from build123d import *

# Parameters (mm, degrees)
EXTRUDE_THIN1_DEPTH = 349.25
FILLET1_R           = 1.016


with BuildPart() as part:
    # Sketch1 → Extrude-Thin1 (new body)
    with BuildSketch(Plane.XY):
        with BuildLine():
            Line((0, 34.925), (-14.2875, 34.925))
            Line((-14.2875, 34.925), (-14.2875, 23.8125))
            Line((-14.2875, 23.8125), (-12.7, 23.8125))
            ThreePointArc((-12.7, 23.8125), (-11.46897023, 18.728780658), (-8.048625, 14.771398298))
            ThreePointArc((-8.048625, 14.771398298), (-4.62827977, 10.814015938), (-3.39725, 5.730296596))
            Line((-3.39725, 5.730296596), (-1.016, 5.730296596))
            Line((-1.016, 5.730296596), (-1.016, 4.7625))
            ThreePointArc((-1.016, 4.7625), (-3.39725, 2.38125), (-1.016, 0))
            Line((-1.016, 0), (0, 0))
            Line((0, 0), (0, 1.016))
            Line((0, 1.016), (-1.016, 1.016))
            ThreePointArc((-1.016, 1.016), (-2.26278514, 2.93751826), (0, 3.29319932))
            Line((0, 3.29319932), (0, 6.746296596))
            Line((0, 6.746296596), (-2.423879893, 6.746296596))
            ThreePointArc((-2.423879893, 6.746296596), (-3.966915161, 11.726057249), (-7.457893571, 15.598013311))
            ThreePointArc((-7.457893571, 15.598013311), (-10.786815308, 19.651741643), (-11.632750432, 24.8285))
            Line((-11.632750432, 24.8285), (-13.2715, 24.8285))
            Line((-13.2715, 24.8285), (-13.2715, 33.909))
            Line((-13.2715, 33.909), (0, 33.909))
            Line((0, 33.909), (0, 34.925))
        make_face()
    extrude(amount=-EXTRUDE_THIN1_DEPTH)

    # Fillet1
    fillet1_edges = [part.edges().sort_by_distance(p)[0] for p in [
        (-11.632750432, 24.8285, -174.625),
        (0, 6.746296596, -174.625),
        (0, 3.29319932, -174.625),
        (-3.39725, 5.730296596, -174.625),
        (-14.2875, 23.8125, -174.625),
        (-14.2875, 34.925, -174.625),
    ]]
    fillet(fillet1_edges, radius=FILLET1_R)


solid = part.part
Build history of the part. All positions in model axes, mm. A direction names the side the tool comes from. Give positions to 0.01 mm unless a question says otherwise; leave off trailing zeros. Write each loop counter-clockwise with the first axis right and the second up, starting at its lowest first coordinate (ties: lowest second). Pieces come first, ordered by that corner, then holes. Notation, with made-up numbers: (35.5, 54.25) - (91.5, 54.25) arc R21 cw to (91.5, 58.25) - close; hole circle Ø8 at (-23.75, 69.5). An arc over 180 degrees is marked (long way). Use one line per item in the form item = value. Start each with the question number.
1. 3-axis set-ups, long thin cutter, end or side, ignore diameter. For faces 5 (the face through (-3.93, 11.66, -172.18)), 6 (the face through (-11.4, 20.1, -349.25)): which of +Z, -Z, +X, -X, +Y, -Y reach the whole face in a straight line?
2. Band-saw the part on B-B on y = 31. Write the cut outline in (x, z).
3. Two-plate mould, pull along Y, no slides. Class faces 1 (the face through (-14.288, 29, -172)), 2 (the face through (-10.535, 19.134, -172.18)), 3 (the face through (-7, 34.925, -172)), 4 (the face through (-13.272, 29, -172)): released by +Y, released by -Y, zero draft, split by the parting line, or undercut.
4. Band-saw the part on A-A on z = -249.5. Write the cut outline in (x, y) (1 decimal).
5. Band-saw the part on C-C on y = 18.5. Write the cut outline in (x, z).
6. Probe line 1 (X direction, y = 32.5, z = -237); line 2 (Y direction, x = -6.5, z = -176) (3 decimals); line 3 (Y direction, x = -5.25, z = -330) (3 decimals). List the from-to ranges inside material, lowest first. Write a range as [from, to].
7. Drop flat-ended pins along their axis: pin 1 Ø3 at (x, y) = (-7, 18.5) entering from -Z; pin 2 Ø1.1 at (y, z) = (5, -225) entering from -X; pin 3 Ø2 at (x, z) = (-12, -178.5) entering from -Y; pin 4 Ø1.5 at (y, z) = (10.5, -215.5) entering from +X. Give the stop position or say it passes through.
Conclusion:
q1.face_5 = +Z, -Z, +X
q1.face_6 = -Z, +X, -X, +Y, -Y
q2.outline = (-14.29, -349.25) - (-13.27, -349.25) - (-13.27, 0) - (-14.29, 0) - close
q3.face_1 = zero draft
q3.face_2 = undercut
q3.face_3 = released by +Y
q3.face_4 = undercut
q4.outline = (-14.3, 24.8) arc R1 ccw to (-13.3, 23.8) - (-12.7, 23.8) arc R11.1 ccw to (-8, 14.8) arc R11.1 cw to (-3.4, 6.7) arc R1 ccw to (-2.4, 5.7) - (-1, 5.7) - (-1, 4.8) arc R2.4 ccw to (-1, 0) - (0, 0) - (0, 1) - (-1, 1) arc R1.4 cw to (-1, 3.7) arc R1 ccw to (0, 4.8) - (0, 5.7) arc R1 ccw to (-1, 6.7) - (-2.4, 6.7) arc R12.1 ccw to (-7.5, 15.6) arc R10.1 cw to (-11.7, 23.8) arc R1 ccw to (-12.7, 24.8) - (-13.3, 24.8) - (-13.3, 33.9) - (0, 33.9) - (0, 34.9) - (-13.3, 34.9) arc R1 ccw to (-14.3, 33.9) - close
q5.outline = (-11.35, -349.25) - (-10.17, -349.25) - (-10.17, 0) - (-11.35, 0) - close
q6.line_1 = [-14.29, -13.27]
q6.line_2 = [13.433, 14.838], [33.909, 34.925]
q6.line_3 = [11.874, 13.563], [33.909, 34.925]
q7.pin_1 = through
q7.pin_2 = -2.2
q7.pin_3 = 17.91
q7.pin_4 = -3.07
